CAD build for the part. Positions are in the model's coordinates, mm. Face numbers are marked on the shaded views. Round coordinates to 2 decimals unless told otherwise and drop trailing zeros. Loops run counter-clockwise (first coordinate to the right, second up) from the corner with the lowest first, then second, coordinate; pieces in that order, holes last. Notation, with made-up numbers: (-32, -39) - (15, -39) arc R33 cw to (15, -2) - close; hole circle Ø3 at (42, 13.5). An arc over 180 degrees is marked (long way). One line per question, with ' | ' between items.
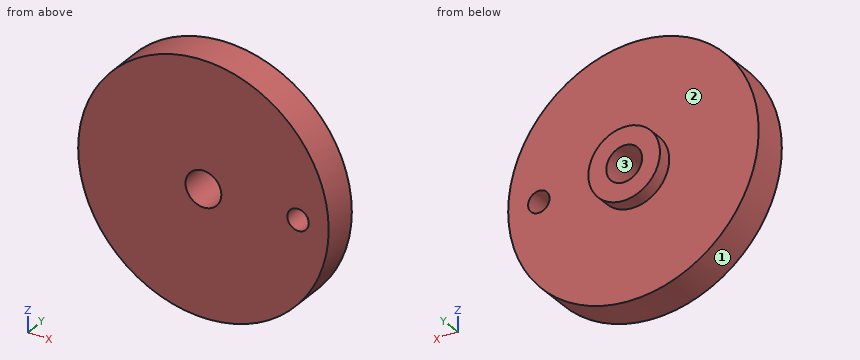
Solid Edge part; units mm, degrees
sketch "Sketch1" plane through (0, 0, 0) normal (0, -1, 0) x (1, 0, 0)
  circle A0 centre (0, 0) radius 17.5
extrude "Protrusion1" add sketch "Sketch1" along normal blind 5
sketch "Sketch2" plane through (0, 0, 0) normal (0, -1, 0) x (1, 0, 0)
  circle A0 centre (0, 0) radius 5
extrude "ExtrudedProtrusion_2" add sketch "Sketch2" against normal blind 2
sketch "Sketch3" plane through (0, 0, 0) normal (0, -1, 0) x (1, 0, 0)
  circle A0 centre (0, 0) radius 2.5
extrude "ExtrudedCutout_3" cut sketch "Sketch3" against normal blind 2
sketch "Sketch4" plane through (0, 0, 0) normal (0, -1, 0) x (1, 0, 0)
  circle A0 centre (0, 0) radius 2.5
extrude "ExtrudedCutout_4" cut sketch "Sketch4" along normal blind 5
sketch "Sketch5" plane through (0, 0, 0) normal (0, -1, 0) x (1, 0, 0)
  circle A0 centre (13.2181, 0) radius 1.5
extrude "ExtrudedCutout_5" cut sketch "Sketch5" along normal blind 5
(1) Cut at A-A, the plane z = 0. Write the cut outline in (x, y), then the cut area to 3 significant figures.
Results found:
outline: (-17.5, -5) - (-2.5, -5) - (-2.5, 2) - (-5, 2) - (-5, 0) - (-17.5, 0) - close; (2.5, -5) - (11.72, -5) - (11.72, 0) - (5, 0) - (5, 2) - (2.5, 2) - close; (14.72, -5) - (17.5, -5) - (17.5, 0) - (14.72, 0) - close | area: 145 mm²
(2) Two-plate mould, pull along X, no slides. Class the marked faces 1, 2 and 3: released by +X, released by -X, zero draft, split by the parting line, or undercut.
Results found:
face 1: split by the parting line | face 2: zero draft | face 3: undercut
(3) Cut at B-B, the plane x = 0. Write the cut outline in (y, z), then the cut area to 3 significant figures.
Results found:
outline: (-5, -17.5) - (0, -17.5) - (0, -5) - (2, -5) - (2, -2.5) - (-5, -2.5) - close; (-5, 2.5) - (2, 2.5) - (2, 5) - (0, 5) - (0, 17.5) - (-5, 17.5) - close | area: 160 mm²
(4) Cut at C-C, the plane y = 1. Write the cut outline in (x, z), then the cut area to 3 significant figures.
Results found:
outline: circle Ø10 at (0, 0); hole circle Ø5 at (0, 0) | area: 58.9 mm²
(5) Cut at D-D, the plane x = 14. Write the cut outline in (y, z), then the cut area to 3 significant figures.
Results found:
outline: (-5, -10.5) - (0, -10.5) - (0, -1.28) - (-5, -1.28) - close; (-5, 1.28) - (0, 1.28) - (0, 10.5) - (-5, 10.5) - close | area: 92.2 mm²
(6) Probe L1, parallel to Z at x = 0, y = 0.75; L2, parallel to Y at x = 15.5, z = 1.5; L3, parallel to Z at x = 0, y = -2. List the from-to ranges inside material, lowest first.
Results found:
L1: z = -5 to -2.5, 2.5 to 5 | L2: y = -5 to 0 | L3: z = -17.5 to -2.5, 2.5 to 17.5
(7) Drop flat-ended pins along their axis: P1, Ø4, axis at y = 1, z = 1.5, coming from the +X side; P2, Ø4, axis at x = -12, y = -3.5, coming from the -Z side; P3, Ø2, axis at x = -2.5, y = -2.5, coming from the +Z side; P4, Ø4, axis at y = -2, z = -12.5, coming from the -X side. Give the stop position or say it passes through.
Results found:
P1: stops at x = 17.5 | P2: stops at z = -14.36 | P3: stops at z = 17.44 | P4: stops at x = -14
